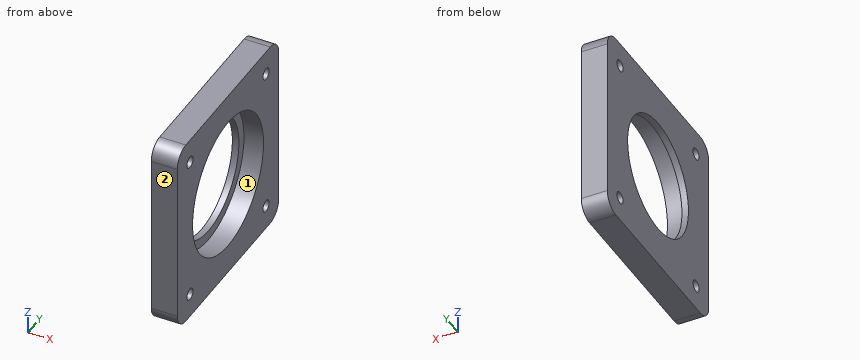
Solid Edge part; units mm, degrees
sketch "Sketch1" plane through (0, 0, 0) normal (1, 0, 0) x (0, 1, 0)
  line L0 (-30, -30) -> (30, -30)
  line L1 (30, -30) -> (30, 30)
  line L2 (30, 30) -> (-30, 30)
  line L3 (-30, 30) -> (-30, -30)
  dimension "D1" = 30
  dimension "D2" = 30
extrude "Protrusion1" add sketch "Sketch1" along normal mid plane 8
hole "Hole_1" at (4, -22.5, 22.5) direction (-1, 0, 0) diameter 3.6 end up to next
hole "Hole1" at (4, 22.5, 22.5) direction (-1, 0, 0) diameter 3.6 end up to next
hole "Hole2" at (4, 22.5, -22.5) direction (-1, 0, 0) diameter 3.6 end up to next
hole "Hole3" at (4, -22.5, -22.5) direction (-1, 0, 0) diameter 3.6 end up to next
hole "Hole_5" at (4, 0, 0) direction (-1, 0, 0) diameter 36 end up to next counterbore diameter 42 counterbore depth 6
fillet "Round_1" radius 5 4 edges at (0, 30, -30) (0, -30, -30) (0, -30, 30) (0, 30, 30)
properties material "Polyethylene, low density"
CAD build for the part. Positions are in the model's coordinates, mm. Face numbers are marked on the shaded views. A direction names the side the tool comes from. Give positions to 0.01 mm unless a question says otherwise; leave off trailing zeros. Write each loop counter-clockwise with the first axis right and the second up, starting at its lowest first coordinate (ties: lowest second). Pieces come first, ordered by that corner, then holes. Notation, with made-up numbers: (-37, 79.25) -> (-1, 79.25) arc R10 ccw to (-1, 83.25) -> close; hole circle Ø1 at (87, 17). An arc over 180 degrees is marked (long way). Return JSON: item names as keys, results as strings.
Item 1: Band-saw the part on A-A (z = 0). List the corners of the cut face in (x, y), then the cut area to 3 significant figures.
Answer below:
{"outline": "(-4, -30) -> (4, -30) -> (4, -21) -> (-2, -21) -> (-2, -18) -> (-4, -18) -> close; (-4, 18) -> (-2, 18) -> (-2, 21) -> (4, 21) -> (4, 30) -> (-4, 30) -> close", "area": "156 mm2"}
Item 2: Band-saw the part on B-B (y = 22.5). List the corners of the cut face in (x, z).
Answer below:
{"outline": "(-4, -30) -> (4, -30) -> (4, -24.3) -> (-4, -24.3) -> close; (-4, -20.7) -> (4, -20.7) -> (4, 20.7) -> (-4, 20.7) -> close; (-4, 24.3) -> (4, 24.3) -> (4, 30) -> (-4, 30) -> close"}
Item 3: Drop flat-ended pins along their axis: pin 1 (4 mm diameter, centred on y = -22.5, z = -22.5, fed in from -X); pin 2 (3 mm diameter, centred on y = 22.5, z = -22.5, fed in from +X). Give the stop position or say it passes through.
Answer below:
{"pin 1": "stops at x = -4", "pin 2": "passes through"}
Item 4: Tool access for the marked faces 1 and 2: list every direction of +Z, -Z, +X, -X, +Y, -Y with a clear straight run to the whole face (end or side of a thin tool).
Answer below:
{"face 1": "+X", "face 2": "+Z, -Z, +X, -X, -Y"}
Item 5: Drill centre lines: probe 1 along Y at (x, z) = (-2.5, 22.5); probe 2 along Z at (x, y) = (-2.5, 0). Where is each one in solid material? Low to high.
Answer below:
{"probe 1": "y = -30 to -24.3, -20.7 to 20.7, 24.3 to 30", "probe 2": "z = -30 to -18, 18 to 30"}
